Autodesk Inventor part; units mm, degrees
ref_plane "YZ Plane" through (0, 0, 0) normal (1, 0, 0) x (0, 1, 0)
ref_plane "XZ Plane" through (0, 0, 0) normal (0, 1, 0) x (-1, 0, 0)
ref_plane "XY Plane" through (0, 0, 0) normal (0, 0, 1) x (1, 0, 0)
sketch "Sketch1" plane through (0, 0, 0) normal (0, 0, 1) x (1, 0, 0)
  line L0 (0, 0) -> (-31.877, 0)
  line L1 (-31.877, 0) -> (-31.877, -5.969)
  line L2 (-31.877, -5.969) -> (0, -5.969)
  line L3 (0, -5.969) -> (0, 0)
  dimension "d0" = 31.877
  dimension "d1" = 5.969
extrude "Extrusion1" add sketch "Sketch1" along normal blind 19.304
shell "Shell1" thickness 1.651 removed faces 1 at (-21.2513, -5.969, 12.8693)
sketch "Sketch2" plane through (-31.877, 0, 0) normal (0, 1, 0) x (1, 0, 0)
  arc A0 (19.8846, -6.604) -> (19.8846, -12.7) centre (13.2486, -9.652) ccw
  arc A1 (0, -7.5459) -> (0, -11.7581) centre (-1.4199, -9.652) ccw
  line L0 (0, 0) -> (0, -19.304)
  line L1 (0, 0) -> (0, -19.304)
  circle A2 centre (-1.4199, -9.652) radius 0.9525
  arc A3 (22.606, -12.7) -> (22.606, -6.604) centre (22.606, -9.652) ccw
  line L2 (31.877, 0) -> (31.877, -19.304)
  line L3 (22.606, -12.7) -> (19.8846, -12.7)
  line L4 (22.606, -6.604) -> (19.8846, -6.604)
  circle A4 centre (-3.175, -17.2678) radius 2.159
  arc A5 (0, -14.5321) -> (0.4881, -19.304) centre (-3.175, -17.2678) ccw
  line L5 (31.877, -19.304) -> (0, -19.304) construction
  line L6 (13.2486, -9.652) -> (-12.5267, -9.652) construction
  circle A6 centre (-3.175, -2.0362) radius 2.159
  arc A7 (0.4881, 0) -> (0, -4.7719) centre (-3.175, -2.0362) ccw
  line L7 (31.877, 0) -> (0, 0)
  line L8 (0, 0) -> (0, -19.304)
  line L9 (31.877, -19.304) -> (0, -19.304)
  line L10 (31.877, 0) -> (31.877, -19.304)
  point P0 (-3.9599, -9.652)
  point P1 (0, -9.652)
  point P2 (5.9461, -9.652)
  point P3 (13.2486, -2.3495)
  point P4 (25.654, -9.652)
  point P5 (-7.366, -17.2678)
  point P6 (-1.4199, -12.192)
  point P7 (-1.4199, -13.462)
  point P8 (0.4881, 0)
  point P9 (0, -4.7719)
  point P10 (0.4881, -19.304)
  point P11 (0, -14.5321)
  dimension "d5" = 14.605
  dimension "d6" = 5.08
  dimension "d8" = 1.905
  dimension "d11" = 9.906
  dimension "d12" = 6.223
  dimension "d13" = 6.096
  dimension "d16" = 4.318
  dimension "d17" = 2.032
  dimension "d18" = 7.366
  dimension "d19" = 1.27
extrude "Extrusion2" add sketch "Sketch2" against normal blind 6.731 contours L0 A1
extrude "Extrusion3" cut sketch "Sketch2" against normal through all contours L4 A3 L3 A0
extrude "Extrusion4" add sketch "Sketch2" against normal blind 1.651 contours A7 L7 L0 | L0 L9 A5
sketch "Sketch3" plane through (0, -5.969, 0) normal (1, 0, 0) x (0, 0, -1)
  line L0 (0, 0) -> (-19.304, 0)
  arc A0 (-7.62, 0) -> (-11.684, 0) centre (-9.652, 0) ccw
  line L1 (0, 0) -> (0, 5.969)
  line L2 (0, 5.969) -> (-19.304, 5.969)
  line L3 (-19.304, 0) -> (-19.304, 5.969)
  line L4 (0, 0) -> (-19.304, 0)
  point P0 (-7.62, 0)
extrude "Extrusion5" cut sketch "Sketch3" against normal up to surface (1.651 mm away) contours L0 A0
ref_plane "Work Plane1" through (-1.27, -5.969, 0) normal (1, 0, 0) x (0, 0, -1)
sketch "Sketch4" plane through (-1.27, -5.969, 0) normal (1, 0, 0) x (0, 0, -1)
  line L0 (0, 4.318) -> (0, 0)
  line L1 (0, 3.81) -> (-2.032, 5.969)
  line L2 (-4.1952, 5.969) -> (0.1228, 5.969)
  line L3 (-2.032, 5.969) -> (0, 5.969)
  line L4 (0, 3.81) -> (0, 5.969)
  line L5 (0, 5.969) -> (-19.304, 5.969) construction
  line L6 (-9.652, 5.969) -> (-9.652, 0) construction
  line L7 (-1.651, 0) -> (-17.653, 0) construction
  line L8 (-19.304, 3.81) -> (-17.272, 5.969)
  line L9 (-19.304, 3.81) -> (-19.304, 5.969)
  line L10 (-19.304, 5.969) -> (-19.304, 4.318)
  line L11 (-19.304, 5.969) -> (-17.272, 5.969)
  dimension "d27" = 3.81
  dimension "d28" = 2.032
extrude "Extrusion6" cut sketch "Sketch4" against normal blind 5.08
sketch "Sketch5" plane through (-31.877, -5.969, 0) normal (0, -1, 0) x (1, 0, 0)
  line L0 (0, 11.7581) -> (0, 19.304)
  line L1 (0, 18.034) -> (0.762, 18.034)
  line L2 (0.762, 18.034) -> (0.762, 15.494)
  line L3 (0.762, 15.494) -> (0, 15.494)
  line L4 (0, 15.494) -> (0, 18.034)
  line L5 (0, 19.304) -> (31.877, 19.304)
  line L6 (0, 7.5459) -> (0, 11.7581) construction
  line L7 (0, 9.652) -> (31.877, 9.652) construction
  line L8 (31.877, 0) -> (31.877, 19.304) construction
  line L9 (0, 1.27) -> (0.762, 1.27)
  line L10 (0.762, 1.27) -> (0.762, 3.81)
  line L11 (0.762, 3.81) -> (0, 3.81)
  line L12 (0, 3.81) -> (0, 1.27)
  point P0 (0, 15.494)
  dimension "d31" = 0.762
  dimension "d32" = 2.54
  dimension "d33" = 1.27
extrude "Extrusion7" cut sketch "Sketch5" against normal up to surface (4.318 mm away)
sketch "Sketch6" plane through (-30.226, -1.651, 1.651) normal (0, -1, 0) x (1, 0, 0)
  circle A0 centre (28.575, 0) radius 0.635
  circle A1 centre (28.575, 0) radius 1.143
  line L0 (28.575, 0) -> (0, 0)
  line L1 (28.575, 5.969) -> (28.575, 0)
  line L2 (30.226, -1.651) -> (30.226, 17.653) construction
  line L3 (30.226, 8.001) -> (-7.0549, 8.001) construction
  circle A2 centre (28.575, 16.002) radius 0.635
  circle A3 centre (28.575, 16.002) radius 1.143
  point P0 (27.432, 0)
  point P1 (28.575, 1.143)
  point P2 (28.575, 0.635)
  point P3 (27.94, 0)
  dimension "d36" = 1.27
  dimension "d37" = 0.508
extrude "Extrusion8" add sketch "Sketch6" along normal up to surface (4.318 mm away) contours A0 L0 A1 L1 | A3 picked at (27.6162, 0.1319)
extrude "Extrusion9" cut sketch "Sketch6" along normal up to surface (4.318 mm away) contours A0 L0 L1 | L1 L0 A0 | A2
properties part number "Back Half Torso" material "Phenolic Resin"
Geometry: final body of the model. Coordinates: model frame, mm. A direction names the side the tool comes from. Give positions to 0.01 mm unless a question says otherwise; leave off trailing zeros. Write each loop counter-clockwise with the first axis right and the second up, starting at its lowest first coordinate (ties: lowest second). Pieces come first, ordered by that corner, then holes. Notation, with made-up numbers: (22, 64) - (50, 64) arc R7 ccw to (50, 72) - close; hole circle Ø11 at (53, 77). An arc over 180 degrees is marked (long way). Return JSON: item names as keys, results as strings. Group by question number.
1) First-contact query: P1, Ø2, axis at y = -3, z = 2.5, coming from the -X side (3 decimals); P2, Ø2, axis at x = -24.5, y = -1.5, coming from the -Z side; P3, Ø8, axis at x = -14.5, z = 10, coming from the -Y side. Flat tips, straight axial feed; report the tip coordinate or a pass-through.
2) Section A-A on x = -13. Return the cut outline in (y, z).
3) Set-up query: faces 5 (the flat face through (-1.27, -1, 19)), 6 (the cylindrical face through (-0.814, -3.937, 9.607)), 7 (the flat face through (-3.774, -1.095, 1.002)), 8 (the flat face through (-30.226, -4, 10)). Return all of +Z, -Z, +X, -X, +Y, -Y with unobstructed straight access to the full face (end or side cutting, diameter ignored); none if empty.
4) Section D-D on z = 0.5. Return the cut outline in (x, y), plus the area to 3 significant figures.
5) Section B-B on y = -5.5. Return the cut outline in (x, z) (1 decimal), plus the area to 3 significant figures.
6) Line query: line 1 (Z direction, x = -26, y = -2.75); line 2 (X direction, y = -2, z = 14); line 3 (Y direction, x = -20.5, z = 0.25). Output: solid intervals per line, ascending.
7) Section C-C on x = -4. Return the cut outline in (y, z).
8) Mould query, pull axis X, two halves, no side actions, for faces 1 (the flat face through (0, -3, 10)), 2 (the flat face through (-37, -1.651, 16)), 3 (the flat face through (-31.115, -4, 17)), 4 (the flat face through (-3.77, -1.09, 18.3)). Classes: released by +X, released by -X, zero draft, split by the parting line, or undercut.
Filled in:
{
 "1": {"P1": "stops at x = -31.115", "P2": "stops at z = 0", "P3": "stops at y = -1.65"},
 "2": {"outline": "(-5.97, 0) - (0, 0) - (0, 5) - (-1.65, 5) - (-1.65, 1.65) - (-5.97, 1.65) - close; (-5.97, 17.65) - (-1.65, 17.65) - (-1.65, 14.3) - (0, 14.3) - (0, 19.3) - (-5.97, 19.3) - close"},
 "3": {"face 5": "+Z, +Y", "face 6": "+X, -Y", "face 7": "-Z, +Y", "face 8": "-Y"},
 "4": {"outline": "(-38.95, -1.65) - (-36.57, -1.65) - (-36.57, 0) - (-38.95, 0) - close; (-33.53, -1.65) - (-31.88, -1.65) - (-31.88, -5.97) - (0, -5.97) - (0, 0) - (-1.27, 0) - (-1.27, -1.63) - (-6.35, -1.63) - (-6.35, 0) - (-33.53, 0) - close", "area": "189 mm^2"},
 "5": {"outline": "(-31.9, 0) - (0, 0) - (0, 7.7) - (-1.7, 7.7) - (-1.7, 2.8) arc R1.1 ccw to (-2.8, 1.7) - (-30.2, 1.7) - (-30.2, 17.7) - (-2.8, 17.7) arc R1.1 ccw to (-1.7, 16.5) - (-1.7, 11.6) - (0, 11.6) - (0, 19.3) - (-31.9, 19.3) - (-31.9, 18) - (-31.1, 18) - (-31.1, 15.5) - (-31.9, 15.5) - (-31.9, 11.8) arc R2.5 ccw (long way) to (-31.9, 7.5) - (-31.9, 3.8) - (-31.1, 3.8) - (-31.1, 1.3) - (-31.9, 1.3) - close; hole circle Ø1.9 at (-33.3, 9.7); hole circle Ø1.3 at (-1.7, 1.7); hole circle Ø1.3 at (-1.7, 17.7)", "area": "161 mm^2"},
 "6": {"line 1": "z = 0 to 1.65, 17.65 to 19.3", "line 2": "x = -31.88 to -30.23, -1.65 to 0", "line 3": "y = -5.97 to 0"},
 "7": {"outline": "(-5.97, 0) - (-2.16, 0) - (0, 2.03) - (0, 17.27) - (-2.16, 19.3) - (-5.97, 19.3) - (-5.97, 17.65) - (-1.65, 17.65) - (-1.65, 1.65) - (-5.97, 1.65) - close"},
 "8": {"face 1": "released by +X", "face 2": "zero draft", "face 3": "released by -X", "face 4": "undercut"}
}
